```python
from build123d import *

# Parameters (mm, degrees)
EXTRUDE_1_DEPTH          = 100
CUT_EXTRUDE_2_DEPTH      = 174.205080757
CUT_EXTRUDE_2_DEPTH_BACK = 174.205080757
SKETCH_2_W               = 40
SKETCH_2_H               = 80
CUT_EXTRUDE_3_DEPTH      = 174.205080757
CUT_EXTRUDE_3_DEPTH_BACK = 174.205080757
SKETCH_3_R               = 2.5
CUT_EXTRUDE_4_DEPTH      = 174.205080757


with BuildPart() as part:
    # 草图1 → 凸台-拉伸1 (new body)
    with BuildSketch(Plane(origin=(0, 0, 0), x_dir=(1, 0, 0), z_dir=(0, 1, 0))):
        Polygon((-50, 100), (50, 100), (100, -100), (-100, -100), align=None)
    extrude(amount=EXTRUDE_1_DEPTH)

    # 草图2 → 切除-拉伸2 (cut, two sides: drawn at the far end of the back side and taken through both)
    with BuildSketch(Plane(origin=(0, 0, 0), x_dir=(0, 0, -1), z_dir=(1, 0, 0)).offset(-CUT_EXTRUDE_2_DEPTH_BACK)):
        with Locations((80, 50)):
            Rectangle(SKETCH_2_W, SKETCH_2_H)
    extrude(amount=CUT_EXTRUDE_2_DEPTH + CUT_EXTRUDE_2_DEPTH_BACK, mode=Mode.SUBTRACT)

    # 草图3 → 切除-拉伸3 (cut, two sides: drawn at the far end of the back side and taken through both)
    with BuildSketch(Plane(origin=(0, 100, 0), x_dir=(1, 0, 0), z_dir=(0, 1, 0)).offset(-CUT_EXTRUDE_3_DEPTH_BACK)):
        with Locations(Location((0, 85, 0), (0, 0, 270))):
            Circle(SKETCH_3_R)
    extrude(amount=CUT_EXTRUDE_3_DEPTH + CUT_EXTRUDE_3_DEPTH_BACK, mode=Mode.SUBTRACT)

    # 草图4 → 切除-拉伸4 (cut, through all)
    with BuildSketch(Plane(origin=(0, 100, 0), x_dir=(1, 0, 0), z_dir=(0, 1, 0))):
        Polygon((-75, 0), (75, 0), (100, -100), (-100, -100), align=None)
    extrude(amount=-CUT_EXTRUDE_4_DEPTH, mode=Mode.SUBTRACT)


solid = part.part
```
Input: part model. Units: mm. Frame: model coordinates. A direction names the side the tool comes from. Coordinates: 2 decimals unless noted, no trailing zeros. Write each loop counter-clockwise with the first axis right and the second up, starting at its lowest first coordinate (ties: lowest second). Pieces come first, ordered by that corner, then holes.
1) Section B-B on z = -85. Output: boundary loops of the cut face in (x, y).
2) Section C-C on y = 8. Output: boundary loops of the cut face in (x, z).
3) Material intervals for line 1 along Z through (x, y) = (0, 4); line 2 along Y through (x, z) = (15.5, -65.5); line 3 along Z through (x, y) = (20.5, 27), sorted ascending.
4) Set-up query: faces 1 (the flat face through (1, 0, -51)), 2 (the flat face through (-1, 10, -80)). Return all of +Z, -Z, +X, -X, +Y, -Y with unobstructed straight access to the full face (end or side cutting, diameter ignored); none if empty.
5) Section A-A on x = 0. Output: boundary loops of the cut face in (y, z), and give its area (3 significant figures).
6) Pin query (flat end, axial travel): pin 1 Ø24 at (x, y) = (8.5, 66.5) entering from -Z; pin 2 Ø10 at (y, z) = (68, -31.5) entering from +X (3 decimals); pin 3 Ø5 at (y, z) = (49, -60.5) entering from +X. Return the tip coordinate at first contact, or that it passes through.
7) Mould query, pull axis X, two halves, no side actions, for faces 3 (the cylindrical face through (0.1, 4.9, -87.5)), 4 (the flat face through (-1, 95, -100)), 5 (the flat face through (65, 49, -40)). Classes: pulls with the +X half, pulls with the -X half, needs draft (parallel to the pull), parting line crosses it, or undercut.
8) Section D-D on x = 33.5. Output: boundary loops of the cut face in (y, z).
Check result:
1. outline: (-53.75, 0) - (-2.5, 0) - (-2.5, 10) - (-53.75, 10) - close; (-53.75, 90) - (-2.5, 90) - (-2.5, 100) - (-53.75, 100) - close; (2.5, 0) - (53.75, 0) - (53.75, 10) - (2.5, 10) - close; (2.5, 90) - (53.75, 90) - (53.75, 100) - (2.5, 100) - close
2. outline: (-75, 0) - (-50, -100) - (50, -100) - (75, 0) - close; hole circle Ø5 at (0, -85)
3. line 1: z = -100 to -87.5, -82.5 to 0
3. line 2: y = 0 to 10, 90 to 100
3. line 3: z = -60 to 0
4. face 1: +Z, -Z, +X, -X, -Y
4. face 2: -Z, +X, -X
5. outline: (0, -100) - (10, -100) - (10, -87.5) - (0, -87.5) - close; (0, -82.5) - (10, -82.5) - (10, -60) - (90, -60) - (90, -82.5) - (100, -82.5) - (100, 0) - (0, 0) - close; (90, -100) - (100, -100) - (100, -87.5) - (90, -87.5) - close
5. area: 6,700 mm2
6. pin 1: stops at z = -60
6. pin 2: stops at x = 68.375
6. pin 3: stops at x = 60.5
7. face 3: undercut
7. face 4: needs draft
7. face 5: pulls with the +X half
8. outline: (0, -100) - (10, -100) - (10, -60) - (90, -60) - (90, -100) - (100, -100) - (100, 0) - (0, 0) - close
